```python
from build123d import *

# Parameters (mm, degrees)
SKETCH_1_R          = 1.75
SKETCH_1_R_2        = 4.25
EXTRUDE_1_DEPTH     = 12
CUT_EXTRUDE_1_DEPTH = 6.5
CUT_EXTRUDE_2_DEPTH = 2.5


with BuildPart() as part:
    # Эскиз1 → Бобышка-Вытянуть1 (new body)
    with BuildSketch(Plane(origin=(0, 0, 0), x_dir=(1, 0, 0), z_dir=(0, 1, 0))):
        with BuildLine():
            Line((5.656854249, -24.04163056), (24.04163056, -5.656854249))
            ThreePointArc((24.04163056, -5.656854249), (26.384776311, 0), (24.04163056, 5.656854249))
            Line((24.04163056, 5.656854249), (5.656854249, 24.04163056))
            ThreePointArc((5.656854249, 24.04163056), (0, 26.384776311), (-5.656854249, 24.04163056))
            Line((-5.656854249, 24.04163056), (-24.04163056, 5.656854249))
            ThreePointArc((-24.04163056, 5.656854249), (-26.384776311, 0), (-24.04163056, -5.656854249))
            Line((-24.04163056, -5.656854249), (-5.656854249, -24.04163056))
            ThreePointArc((-5.656854249, -24.04163056), (0, -26.384776311), (5.656854249, -24.04163056))
        make_face()
        with Locations(Location((21.213203436, 0, 0), (0, 0, 270))):
            Circle(SKETCH_1_R, mode=Mode.SUBTRACT)
        with Locations(Location((0, -21.213203436, 0), (0, 0, 270))):
            Circle(SKETCH_1_R, mode=Mode.SUBTRACT)
        with Locations(Location((-21.213203436, 0, 0), (0, 0, 270))):
            Circle(SKETCH_1_R, mode=Mode.SUBTRACT)
        with Locations(Location((0, 21.213203436, 0), (0, 0, 270))):
            Circle(SKETCH_1_R, mode=Mode.SUBTRACT)
        with Locations(Location((0, 0, 0), (0, 0, 270))):
            Circle(SKETCH_1_R_2, mode=Mode.SUBTRACT)
    extrude(amount=EXTRUDE_1_DEPTH)

    # Эскиз2 → Вырез-Вытянуть1 (cut)
    with BuildSketch(Plane(origin=(0, 12, 0), x_dir=(1, 0, 0), z_dir=(0, 1, 0))):
        Polygon((3.781644263, -6.55), (7.563288526, 0), (3.781644263, 6.55), (-3.781644263, 6.55), (-7.563288526, 0), (-3.781644263, -6.55), align=None)
    extrude(amount=-CUT_EXTRUDE_1_DEPTH, mode=Mode.SUBTRACT)

    # Эскиз4 → Вырез-Вытянуть2 (cut)
    with BuildSketch(Plane.XZ):
        Polygon((24.063203436, -1.645448267), (24.063203436, 1.645448267), (21.213203436, 3.290896534), (18.363203436, 1.645448267), (18.363203436, -1.645448267), (21.213203436, -3.290896534), align=None)
        Polygon((-1.645448267, 18.363203436), (1.645448267, 18.363203436), (3.290896534, 21.213203436), (1.645448267, 24.063203436), (-1.645448267, 24.063203436), (-3.290896534, 21.213203436), align=None)
        Polygon((-1.645448267, -24.063203436), (1.645448267, -24.063203436), (3.290896534, -21.213203436), (1.645448267, -18.363203436), (-1.645448267, -18.363203436), (-3.290896534, -21.213203436), align=None)
        Polygon((-24.063203436, 1.645448267), (-24.063203436, -1.645448267), (-21.213203436, -3.290896534), (-18.363203436, -1.645448267), (-18.363203436, 1.645448267), (-21.213203436, 3.290896534), align=None)
    extrude(amount=-CUT_EXTRUDE_2_DEPTH, mode=Mode.SUBTRACT)


solid = part.part
```
The model under review builds one solid part; all positions refer to its coordinate system, in mm. A direction names the side the tool comes from. Round coordinates to 2 decimals unless told otherwise and drop trailing zeros. Order: outer loops, then holes, each group sorted by start corner. A loop starts at its lowest first (then second) coordinate and runs counter-clockwise, first axis right, second up. Notation, with made-up numbers: (0, 68) -> (34, 68) arc R4 cw to (34, 75) -> close; hole circle Ø6 at (31, 86.25). An arc over 180 degrees is marked (long way). One line per item, written item: value. Start each with the question number.
Q1. Take a section at A-A (x = 0). Write out the cut boundary in (y, z), and give its area (3 significant figures).
Q2. Machinability: for faces 4 (the face through (0, 1, 18.363)), 5 (the face through (3.3, 5.5, -3)), 6 (the face through (14.7, 5.9, 15)), which of the approach directions +Z, -Z, +X, -X, +Y, -Y give a long, thin tool a straight path to every point of the face, cutting with its end or side? Answer none if there is none.
Q3. Mouldability with a two-part tool opening along Z and no side actions: class faces 1 (the face through (0, 0, 5)), 2 (the face through (-22.658, 1.232, -2.457)), 3 (the face through (-14.7, 5.9, -15)) as released by +Z, released by -Z, zero draft, split by the parting line, or undercut.
Q4. Wall thickness on line 1 (Z direction, x = 0, y = 10.75); line 2 (Z direction, x = 0, y = 2.4); line 3 (X direction, y = 3.75, z = 0): over which ranges is each line inside the solid? List them lowest first.
Q5. Take a section at D-D (x = -17.5). Write out the cut boundary in (y, z).
Q6. Clearance check with flat-ended pins moving along their axes: pin 1 Ø1.7 at (x, z) = (1.5, -22) entering from -Y; pin 2 Ø1.2 at (x, y) = (1, 1.5) entering from +Z; pin 3 Ø1.5 at (x, y) = (-19, 5.5) entering from +Z. State where each tip first meets the part, or that it passes through.
Q7. Take a section at C-C (y = 1). Count the separate pieces of the cut face and the enclosed holes in it, and give its area (3 significant figures).
Q8. Take a section at B-B (y = 6.75). Write out the cut boundary in (x, z).
Reported:
1. outline: (0, -26.38) -> (12, -26.38) -> (12, -22.96) -> (2.5, -22.96) -> (2.5, -24.06) -> (0, -24.06) -> close; (0, -18.36) -> (2.5, -18.36) -> (2.5, -19.46) -> (12, -19.46) -> (12, -6.55) -> (5.5, -6.55) -> (5.5, -4.25) -> (0, -4.25) -> close; (0, 4.25) -> (5.5, 4.25) -> (5.5, 6.55) -> (12, 6.55) -> (12, 19.46) -> (2.5, 19.46) -> (2.5, 18.36) -> (0, 18.36) -> close; (0, 24.06) -> (2.5, 24.06) -> (2.5, 22.96) -> (12, 22.96) -> (12, 26.38) -> (0, 26.38) -> close
1. area: 406 mm2
2. face 4: -Y
2. face 5: +Y
2. face 6: +Z, +X, +Y, -Y
3. face 1: zero draft
3. face 2: undercut
3. face 3: released by -Z
4. line 1: z = -26.38 to -22.96, -19.46 to -6.55, 6.55 to 19.46, 22.96 to 26.38
4. line 2: z = -26.38 to -24.06, -18.36 to -4.25, 4.25 to 18.36, 24.06 to 26.38
4. line 3: x = -26.38 to -22.96, -19.46 to -4.25, 4.25 to 19.46, 22.96 to 26.38
5. outline: (0, -12.2) -> (12, -12.2) -> (12, 12.2) -> (0, 12.2) -> close
6. pin 1: stops at y = 2.5
6. pin 2: stops at z = 26.37
6. pin 3: stops at z = 11.45
7. separate pieces: 1
7. enclosed holes: 5
7. area: 1,540 mm2
8. outline: (-24.04, -5.66) -> (-5.66, -24.04) arc R8 ccw to (5.66, -24.04) -> (24.04, -5.66) arc R8 ccw to (24.04, 5.66) -> (5.66, 24.04) arc R8 ccw to (-5.66, 24.04) -> (-24.04, 5.66) arc R8 ccw to start; hole circle Ø3.5 at (-21.21, 0); hole (-7.56, 0) -> (-3.78, -6.55) -> (3.78, -6.55) -> (7.56, 0) -> (3.78, 6.55) -> (-3.78, 6.55) -> close; hole circle Ø3.5 at (0, -21.21); hole circle Ø3.5 at (0, 21.21); hole circle Ø3.5 at (21.21, 0)
